Design review of the part built by this model. Coordinates are the model's own, in mm. A direction names the side the tool comes from. Give positions to 0.01 mm unless a question says otherwise; leave off trailing zeros. Write each loop counter-clockwise with the first axis right and the second up, starting at its lowest first coordinate (ties: lowest second). Pieces come first, ordered by that corner, then holes. Notation, with made-up numbers: (20, 73.5) - (46, 73.5) arc R21 ccw to (46, 106.5) - close; hole circle Ø1 at (-26.75, 8). An arc over 180 degrees is marked (long way). Use a Markdown table: item, result. Add a question column.
```python
from build123d import *

# Parameters (mm, degrees)
SKETCH1_W         = 12.7
SKETCH1_H         = 177.8
EXTRUSION1_DEPTH  = 20.574
EXTRUSION3_DEPTH  = 20.32
SKETCH4_R         = 6.35
EXTRUSION4_DEPTH  = 20.32
EXTRUSION5_DEPTH  = 0.254
SKETCH7_R         = 6.0071
EXTRUSION7_DEPTH  = 0.508
SKETCH8_R         = 4.826
EXTRUSION8_DEPTH  = 22.86
SKETCH9_R         = 8.89
SKETCH9_R_2       = 6.0071
EXTRUSION9_DEPTH  = 16.002
SKETCH10_R        = 6.0071
SKETCH10_R_2      = 4.826
EXTRUSION10_DEPTH = 16.002
SKETCH11_W        = 12.7
SKETCH11_H        = 20.574
EXTRUSION14_DEPTH = 25.4
SKETCH12_W        = 25.4
SKETCH12_H        = 20.574
EXTRUSION15_DEPTH = 2.54


with BuildPart() as part:
    # Sketch1 → Extrusion1 (new body)
    with BuildSketch(Plane(origin=(0, 0, 0), x_dir=(-1, 0, 0), z_dir=(0, 1, 0))):
        with Locations((6.35, -88.9)):
            Rectangle(SKETCH1_W, SKETCH1_H)
    extrude(amount=EXTRUSION1_DEPTH)

    # Sketch3 → Extrusion3 (add)
    with BuildSketch(Plane.XZ):
        Polygon((-12.7, -152.4), (-12.7, -146.7612), (-86.303547963, -127.039188763), (-86.303547963, -73.699188763), (-93.415547963, -73.699188763), (-93.415547963, -127.039188763), (-87.713247963, -132.300260787), align=None)
    extrude(amount=-EXTRUSION3_DEPTH)

    # Sketch4 → Extrusion4 (cut)
    with BuildSketch(Plane.ZY.offset(12.7)):
        with Locations((-12.7, 10.287)):
            Circle(SKETCH4_R)
    extrude(amount=-EXTRUSION4_DEPTH, mode=Mode.SUBTRACT)

    # Sketch5 → Extrusion5 (add)
    with BuildSketch(Plane(origin=(0, 20.32, 0), x_dir=(1, 0, 0), z_dir=(0, 1, 0))):
        Polygon((-86.303547963, 73.699188763), (-86.303547963, 127.039188763), (-12.7, 146.7612), (-12.7, 152.4), (-87.713247963, 132.300260787), (-93.415547963, 127.039188763), (-93.415547963, 73.699188763), align=None)
    extrude(amount=EXTRUSION5_DEPTH)

    # Sketch7 → Extrusion7 (cut)
    with BuildSketch(Plane.ZY.offset(93.415547963)):
        with Locations((-83.770288763, 10.287)):
            Circle(SKETCH7_R)
    extrude(amount=-EXTRUSION7_DEPTH, mode=Mode.SUBTRACT)

    # Sketch8 → Extrusion8 (cut)
    with BuildSketch(Plane.ZY.offset(92.907547963)):
        with Locations((-83.770288763, 10.287)):
            Circle(SKETCH8_R)
    extrude(amount=-EXTRUSION8_DEPTH, mode=Mode.SUBTRACT)

    # Sketch9 → Extrusion9 (add)
    with BuildSketch(Plane(origin=(-86.303547963, 0, 0), x_dir=(0, 0, -1), z_dir=(1, 0, 0))):
        with Locations((83.770288763, 10.287)):
            Circle(SKETCH9_R)
        with Locations((83.770288763, 10.287)):
            Circle(SKETCH9_R_2, mode=Mode.SUBTRACT)
    extrude(amount=EXTRUSION9_DEPTH)

    # Sketch10 → Extrusion10 (add)
    with BuildSketch(Plane(origin=(-86.303547963, 10.287, -83.770288763), x_dir=(0, 0, -1), z_dir=(1, 0, 0))):
        Circle(SKETCH10_R)
        Circle(SKETCH10_R_2, mode=Mode.SUBTRACT)
    extrude(amount=EXTRUSION10_DEPTH)

    # Sketch11 → Extrusion14 (add)
    with BuildSketch(Plane(origin=(0, 0, -177.8), x_dir=(-1, 0, 0), z_dir=(0, 0, -1))):
        with Locations((6.35, 10.287)):
            Rectangle(SKETCH11_W, SKETCH11_H)
    extrude(amount=EXTRUSION14_DEPTH)

    # Sketch12 → Extrusion15 (add)
    with BuildSketch(Plane.ZY.offset(12.7)):
        with Locations((-190.5, 10.287)):
            Rectangle(SKETCH12_W, SKETCH12_H)
    extrude(amount=EXTRUSION15_DEPTH)


solid = part.part
```
(1) Mouldability with a two-part tool opening along Z and no side actions: class faces 6 (the face through (-12, 0, -110)), 7 (the face through (-8, 10, -203.2)), 8 (the face through (-93.17, 12.09, -78.04)), 9 (the face through (-90, 10, -73.699)) as +Z half, -Z half, draft (parallel to the pull), parting line (faces both ways), or undercut.
(2) Add section C-C (x = -78.5). State the section outline as (y, z) points.
(3) Add section D-D (z = -184). State the section outline as (x, y) points, and give its area (3 significant figures).
(4) Tool access review of faces 1 (the face through (-12.7, 10, -165)), 2 (the face through (-15.24, 10, -191)), 3 (the face through (-92.908, 15.2, -82.9)), 4 (the face through (-50.02, 10.14, -136.76)), 5 (the face through (-78.41, 12.96, -92.25)): name each direction out of +Z, -Z, +X, -X, +Y, -Y from which nothing blocks a thin tool from reaching the whole face with its end or side.
(5) Add section A-A (z = -12.7). State the section outline as (x, y) points, and give its area (4 significant figures).
(6) Add section B-B (y = 13). Count the separate pieces of the cut face and the enclosed holes in it, and give its area (3 significant figures).
(7) Insertion check: pin 1 (2 mm diameter, centred on x = -14, y = 10.5, fed in from +Z); pin 2 (1 mm diameter, centred on x = -30.5, y = 14, fed in from +Z); pin 3 (1.5 mm diameter, centred on y = 18.5, z = -47.5, fed in from -X); pin 4 (11.5 mm diameter, centred on y = 10.287, z = -12.7, fed in from -X). Each pin has a flat end and moves straight along its axis. Give the tip position at first contact, or say it passes through.
(8) For line 1 along Y through (x, z) = (-5.75, -12.7); line 2 along Z through (x, y) = (-71, 13.25); line 3 along X through (y, z) = (16.5, -101.5), list the stretches that pass through material, from the lowest coordinate up.
Answers follow:
| question | item | result |
|---|---|---|
| 1 | face 6 | draft |
| 1 | face 7 | -Z half |
| 1 | face 8 | undercut |
| 1 | face 9 | +Z half |
| 2 | outline | (0, -134.77) - (20.57, -134.77) - (20.57, -129.13) - (0, -129.13) - close; circle Ø17.78 at (10.29, -83.77); hole circle Ø9.65 at (10.29, -83.77) |
| 3 | outline | (-15.24, 0) - (0, 0) - (0, 20.57) - (-15.24, 20.57) - close |
| 3 | area | 314 mm^2 |
| 4 | face 1 | -X, +Y, -Y |
| 4 | face 2 | -Z, -X, +Y, -Y |
| 4 | face 3 | -X |
| 4 | face 4 | +Y, -Y |
| 4 | face 5 | none |
| 5 | outline | (-12.7, 0) - (0, 0) - (0, 3.94) - (-12.7, 3.94) - close; (-12.7, 16.64) - (0, 16.64) - (0, 20.57) - (-12.7, 20.57) - close |
| 5 | area | 100.0 mm^2 |
| 6 | separate pieces | 3 |
| 6 | enclosed holes | 0 |
| 6 | area | 3,400 mm^2 |
| 7 | pin 1 | z = -146.14 |
| 7 | pin 2 | z = -141.86 |
| 7 | pin 3 | x = -12.7 |
| 7 | pin 4 | through |
| 8 | line 1 | 0 to 3.94, 16.64 to 20.57 |
| 8 | line 2 | -136.78 to -131.14, -92.15 to -87.58, -79.96 to -75.39 |
| 8 | line 3 | -93.42 to -86.3, -12.7 to 0 |
